Work out the finished part from the listing and answer in its coordinate system (mm). A direction names the side the tool comes from. Coordinates: 2 decimals unless noted, no trailing zeros. Order: outer loops, then holes, each group sorted by start corner. A loop starts at its lowest first (then second) coordinate and runs counter-clockwise, first axis right, second up. Notation, with made-up numbers: M 11.25,59 L 17.25,59 A20 ccw 17.25,89 Z; hole C 16.25,3.25 d5. An arc over 180 degrees is marked long. Use a Markdown table: item, result.
from build123d import *

# Parameters (mm, degrees)
SKETCH_1_W      = 30
SKETCH_1_H      = 30
SKETCH_1_R      = 1.6
EXTRUDE_1_DEPTH = 5
SKETCH_2_W      = 9.6
SKETCH_2_H      = 30
EXTRUDE_2_DEPTH = 0.3
CHAMFER_2_SIZE  = 0.3


with BuildPart() as part:
    # 草图1 → 凸台-拉伸1 (new body)
    with BuildSketch(Plane(origin=(0, 0, 0), x_dir=(1, 0, 0), z_dir=(0, 1, 0))):
        with Locations((15, -15)):
            Rectangle(SKETCH_1_W, SKETCH_1_H)
        with Locations(Location((7.5, -7, 0), (0, 0, 270))):
            Circle(SKETCH_1_R, mode=Mode.SUBTRACT)
        with Locations(Location((22.5, -7, 0), (0, 0, 270))):
            Circle(SKETCH_1_R, mode=Mode.SUBTRACT)
        with Locations(Location((22.5, -23, 0), (0, 0, 270))):
            Circle(SKETCH_1_R, mode=Mode.SUBTRACT)
        with Locations(Location((7.5, -23, 0), (0, 0, 270))):
            Circle(SKETCH_1_R, mode=Mode.SUBTRACT)
    extrude(amount=EXTRUDE_1_DEPTH)

    # 草图2 → 凸台-拉伸2 (add)
    with BuildSketch(Plane(origin=(0, 5, 0), x_dir=(1, 0, 0), z_dir=(0, 1, 0))):
        with Locations((15, -15)):
            Rectangle(SKETCH_2_W, SKETCH_2_H)
    extrude(amount=EXTRUDE_2_DEPTH)

    # 倒角2
    chamfer_2_edges = [part.edges().sort_by_distance(p)[0] for p in [
        (19.8, 5.3, 15),
        (10.2, 5.3, 15),
    ]]
    chamfer(chamfer_2_edges, length=CHAMFER_2_SIZE - 0.0001)  # a hair under: the kernel refuses the full size


solid = part.part
1. For a pull along X with two mould halves and no side action, classify faces 1 (the face through (0, 2, 15)), 2 (the face through (6.08, 2.46, 23.74)), 3 (the face through (5.94, 2.46, 6.65)), 4 (the face through (15, 3, 30)) as +X half, -X half, draft (parallel to the pull), parting line (faces both ways), or undercut.
Answers below:
| item | result |
|---|---|
| face 1 | -X half |
| face 2 | undercut |
| face 3 | undercut |
| face 4 | draft |
2. Section A-A on x = 7.5 is taken. Determine the outline of the cut face in (y, z).
Answers below:
| item | result |
|---|---|
| outline | M 0,0 L 5,0 L 5,5.4 L 0,5.4 Z; M 0,8.6 L 5,8.6 L 5,21.4 L 0,21.4 Z; M 0,24.6 L 5,24.6 L 5,30 L 0,30 Z |
3. Section B-B on z = 23 is taken. Give the number of separate pieces and of enclosed holes in the cut face, then the cut area to 3 significant figures.
Answers below:
| item | result |
|---|---|
| separate pieces | 3 |
| enclosed holes | 0 |
| area | 121 mm² |
4. For faces 5 (the face through (5, 5, 15)), 6 (the face through (15, 0, 15)), 7 (the face through (25, 5, 15)), determine the directions among +Z, -Z, +X, -X, +Y, -Y from which every point of the face is accessible in a straight line to the end or side of a thin tool.
Answers below:
| item | result |
|---|---|
| face 5 | +Z, -Z, -X, +Y |
| face 6 | +Z, -Z, +X, -X, -Y |
| face 7 | +Z, -Z, +X, +Y |
5. Find the intervals of material crossed by probe 1 along X at (y, z) = (2.65, 23); probe 2 along X at (y, z) = (1, 8); probe 3 along Y at (x, z) = (26.5, 22.25), in increasing order.
Answers below:
| item | result |
|---|---|
| probe 1 | 0 to 5.9, 9.1 to 20.9, 24.1 to 30 |
| probe 2 | 0 to 6.25, 8.75 to 21.25, 23.75 to 30 |
| probe 3 | 0 to 5 |
6. Flat-ended cylindrical pins translate along their axes: P1, Ø2.5, axis at x = 22.5, z = 7, coming from the -Y side; P2, Ø1, axis at x = 5, z = 7, coming from the +Y side. Find the tip coordinate at first contact, or state that the pin passes through.
Answers below:
| item | result |
|---|---|
| P1 | through |
| P2 | y = 5 |
7. Section C-C on y = 3.05 is taken. Determine the outline of the cut face in (x, z).
Answers below:
| item | result |
|---|---|
| outline | M 0,0 L 30,0 L 30,30 L 0,30 Z; hole C 7.5,7 d3.2; hole C 7.5,23 d3.2; hole C 22.5,7 d3.2; hole C 22.5,23 d3.2 |
